```python
from build123d import *

# Parameters (mm, degrees)
BOSS_EXTRUDE1_DEPTH                               = 6.35
F_7_0_201_DIAMETER_HOLE1_D                        = 5.1054
CIRPATTERN1_COUNT                                 = 2
CSK_FOR_8_FLAT_HEAD_MACHINE_SCREW_100_D           = 4.3053
CSK_FOR_8_FLAT_HEAD_MACHINE_SCREW_100_CSINK_D     = 8.4328
CSK_FOR_8_FLAT_HEAD_MACHINE_SCREW_100_CSINK_ANGLE = 100
CIRPATTERN2_COUNT                                 = 8


with BuildPart() as part:
    # Sketch1 → Boss-Extrude1 (new body)
    with BuildSketch(Plane(origin=(0, 0, 0), x_dir=(1, 0, 0), z_dir=(0, 1, 0))):
        Polygon((-92.075, 46.99), (-44.45, 94.615), (44.45, 94.615), (92.075, 46.99), (92.075, -46.99), (44.45, -94.615), (-44.45, -94.615), (-92.075, -46.99), align=None)
    extrude(amount=BOSS_EXTRUDE1_DEPTH)

    # #7 (0.201) Diameter Hole1 (through all)
    with Locations(Plane(origin=(0, 6.35, 0), x_dir=(-1, 0, 0), z_dir=(0, 1, 0))):
        with Locations((36.5125, -67.31), (-36.5125, -67.31)):
            f_7_0_201_diameter_hole1 = Hole(F_7_0_201_DIAMETER_HOLE1_D / 2)

    # CirPattern1: #7 (0.201) Diameter Hole1 ×2 about axis
    cirpattern1_axis = Axis((0, 0, 0), (0, 1, 0))
    for i in range(1, CIRPATTERN1_COUNT):
        add(f_7_0_201_diameter_hole1.rotate(cirpattern1_axis, i * 360 / CIRPATTERN1_COUNT), mode=Mode.SUBTRACT)

    # CSK for #8 Flat Head Machine Screw (100)1 (through all)
    with Locations(Plane(origin=(0, 6.35, 0), x_dir=(-1, 0, 0), z_dir=(0, 1, 0))):
        with Locations((0, 31.75)):
            csk_for_8_flat_head_machine_screw_100 = CounterSinkHole(CSK_FOR_8_FLAT_HEAD_MACHINE_SCREW_100_D / 2, CSK_FOR_8_FLAT_HEAD_MACHINE_SCREW_100_CSINK_D / 2, counter_sink_angle=CSK_FOR_8_FLAT_HEAD_MACHINE_SCREW_100_CSINK_ANGLE)

    # CirPattern2: CSK for #8 Flat Head Machine Screw (100)1 ×8 about axis
    cirpattern2_axis = Axis((0, 0, 0), (0, 1, 0))
    for i in range(1, CIRPATTERN2_COUNT):
        add(csk_for_8_flat_head_machine_screw_100.rotate(cirpattern2_axis, i * 360 / CIRPATTERN2_COUNT), mode=Mode.SUBTRACT)


solid = part.part
```
Geometry: final body of the model. Coordinates: model frame, mm. Coordinates: 2 decimals unless noted, no trailing zeros. Order: outer loops, then holes, each group sorted by start corner. A loop starts at its lowest first (then second) coordinate and runs counter-clockwise, first axis right, second up. Notation, with made-up numbers: (69, -28.5) -> (96, -28.5) arc R26 cw to (96, -6.5) -> close; hole circle Ø7 at (25, 79.25). An arc over 180 degrees is marked (long way). Answer in a Markdown table with one row per item.
Item 1: Section C-C on z = 31.75. Output: boundary loops of the cut face in (x, y) (3 decimals).
Return value:
| item | result |
|---|---|
| outline | (-92.075, 0) -> (-2.153, 0) -> (-2.153, 4.618) -> (-4.216, 6.35) -> (-92.075, 6.35) -> close; (2.153, 0) -> (92.075, 0) -> (92.075, 6.35) -> (4.216, 6.35) -> (2.153, 4.618) -> close |
Item 2: Draft query along X for faces 1 (the cylindrical face through (-33.884, 2.277, -0.28)), 2 (the cylindrical face through (-36.18, 3.13, 64.78)), 3 (the flat face through (-92.075, 3, 1)), 4 (the flat face through (1, 0, -1)). Return one class per face: released by +X, released by -X, zero draft, split by the parting line, or undercut.
Return value:
| item | result |
|---|---|
| face 1 | undercut |
| face 2 | undercut |
| face 3 | released by -X |
| face 4 | zero draft |
Item 3: Section A-A on z = 0. Output: boundary loops of the cut face in (x, y) (3 decimals), plus the area to 3 significant figures.
Return value:
| item | result |
|---|---|
| outline | (-92.075, 0) -> (-33.903, 0) -> (-33.903, 4.618) -> (-35.966, 6.35) -> (-92.075, 6.35) -> close; (-29.597, 0) -> (29.597, 0) -> (29.597, 4.618) -> (27.534, 6.35) -> (-27.534, 6.35) -> (-29.597, 4.618) -> close; (33.903, 0) -> (92.075, 0) -> (92.075, 6.35) -> (35.966, 6.35) -> (33.903, 4.618) -> close |
| area | 1,110 mm² |
Item 4: Section D-D on x = -31.75. Output: boundary loops of the cut face in (y, z) (3 decimals), plus the area to 3 significant figures.
Return value:
| item | result |
|---|---|
| outline | (0, -94.615) -> (6.35, -94.615) -> (6.35, -4.216) -> (4.618, -2.153) -> (0, -2.153) -> close; (0, 2.153) -> (4.618, 2.153) -> (6.35, 4.216) -> (6.35, 94.615) -> (0, 94.615) -> close |
| area | 1,170 mm² |
Item 5: Ray query, L1, parallel to X at y = 2.7, z = 31.75 (3 decimals); L2, parallel to X at y = 3.75, z = 0 (3 decimals); L3, parallel to Z at x = 31.75, y = 2.9 (3 decimals). Return the intervals inside material, ascending.
Return value:
| item | result |
|---|---|
| L1 | x = -92.075 to -2.153, 2.153 to 92.075 |
| L2 | x = -92.075 to -33.903, -29.597 to 29.597, 33.903 to 92.075 |
| L3 | z = -94.615 to -2.153, 2.153 to 94.615 |
Item 6: Section B-B on x = 0. Output: boundary loops of the cut face in (y, z) (3 decimals).
Return value:
| item | result |
|---|---|
| outline | (0, -94.615) -> (6.35, -94.615) -> (6.35, -35.966) -> (4.618, -33.903) -> (0, -33.903) -> close; (0, -29.597) -> (4.618, -29.597) -> (6.35, -27.534) -> (6.35, 27.534) -> (4.618, 29.597) -> (0, 29.597) -> close; (0, 33.903) -> (4.618, 33.903) -> (6.35, 35.966) -> (6.35, 94.615) -> (0, 94.615) -> close |
Item 7: Contact query for flat-ended pins moving along their axis: P1, Ø5, axis at x = -22.45, z = 22.45, coming from the +Y side; P2, Ø7, axis at x = -22.45, z = -22.45, coming from the +Y side; P3, Ø2, axis at x = -66, y = 1, coming from the -Z side (3 decimals). Output: stop coordinate, or through.
Return value:
| item | result |
|---|---|
| P1 | stops at y = 4.91 |
| P2 | stops at y = 5.75 |
| P3 | stops at z = -74.065 |
